```python
from build123d import *

# Parameters (mm, degrees)
SKETCH_2_R      = 1.25
EXTRUDE_1_DEPTH = 1.8


with BuildPart() as part:
    # Эскиз2 → Бобышка-Вытянуть1 (new body)
    with BuildSketch(Plane(origin=(0, 0, 0), x_dir=(1, 0, 0), z_dir=(0, 1, 0))):
        with Locations(Location((0, 0, 0), (0, 0, 270))):
            Circle(SKETCH_2_R)
    extrude(amount=-EXTRUDE_1_DEPTH)

    # Эскиз4 → Повернуть1 (revolve)
    with BuildSketch(Plane.XY, mode=Mode.PRIVATE) as revolve_1_sk:
        with BuildLine():
            Line((0, 0), (0, 1))
            Line((0, 1), (4, 1))
            ThreePointArc((4, 1), (3.323810781, 0.850092459), (2.774328891, 0.428460175))
            Line((2.774328891, 0.428460175), (2.654597544, 0.285769912))
            ThreePointArc((2.654597544, 0.285769912), (2.379856599, 0.07495377), (2.041761989, 0))
            Line((2.041761989, 0), (1.25, 0))
            Line((1.25, 0), (0, 0))
        make_face()
    revolve(revolve_1_sk.sketch.rotate(Axis((0, 0, 0), (0, 1, 0)), 90), axis=Axis((0, 0, 0), (0, 1, 0)))


solid = part.part
```
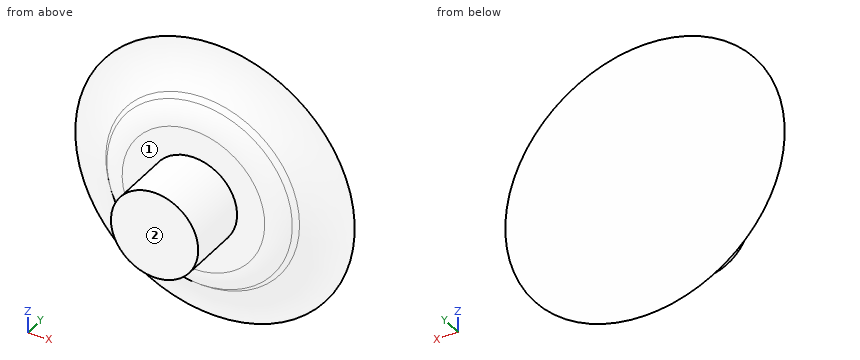
Work out the finished part from the listing and answer in its coordinate system (mm). Face numbers are marked on the shaded views. A direction names the side the tool comes from. Give positions to 0.01 mm unless a question says otherwise; leave off trailing zeros. Order: outer loops, then holes, each group sorted by start corner. A loop starts at its lowest first (then second) coordinate and runs counter-clockwise, first axis right, second up. Notation, with made-up numbers: (79, -27) -> (131, -27) arc R18 ccw to (131, 6) -> close; hole circle Ø2 at (-28.75, -16). An arc over 180 degrees is marked (long way). Answer as CSV lines item,"result". Start each with the question number.
(1) Section B-B, the plane z = 0 is taken. Write down the section's boundary in (x, y), plus the area to 3 significant figures.
(2) This flat-tipped pin is pushed along its axis until it touches: pin 1 Ø1.5 at (y, z) = (-1, -1.5) entering from -X. Where does it stop, or does it pass through?
(3) Which of the six approach directions +Z, -Z, +X, -X, +Y, -Y give full straight-line access (tool end or side, diameter ignored) to the marked faces 1 and 2?
(4) Section A-A, the plane x = 0 is taken. Write down the section's boundary in (y, z), plus the area to 3 significant figures.
(5) Section C-C, the plane y = 0.7 is taken. Write down the section's boundary in (x, z), plus the area to 3 significant figures.
(6) Section D-D, the plane y = -0.3 is taken. Write down the section's boundary in (x, z), plus the area to 3 significant figures.
(7) Consider line 1 along Z through (x, y) = (1.25, 0.6); line 2 along Y through (x, z) = (0.25, -3); line 3 along Z through (x, y) = (-1, 0.6). Determine where each line is inside the solid, lowest interval first.
Entries:
1,outline,"(-4, 1) arc R1.6 cw to (-2.77, 0.43) -> (-2.65, 0.29) arc R0.8 ccw to (-2.04, 0) -> (-1.25, 0) -> (-1.25, -1.8) -> (1.25, -1.8) -> (1.25, 0) -> (2.04, 0) arc R0.8 ccw to (2.65, 0.29) -> (2.77, 0.43) arc R1.6 cw to (4, 1) -> close"
1,area,"10.3 mm²"
2,pin 1,"x = -1"
3,face 1,"-Y"
3,face 2,"+Z, -Z, +X, -X, -Y"
4,outline,"(-1.8, -1.25) -> (0, -1.25) -> (0, -2.04) arc R0.8 ccw to (0.29, -2.65) -> (0.43, -2.77) arc R1.6 cw to (1, -4) -> (1, 4) arc R1.6 cw to (0.43, 2.77) -> (0.29, 2.65) arc R0.8 ccw to (0, 2.04) -> (0, 1.25) -> (-1.8, 1.25) -> close"
4,area,"10.3 mm²"
5,outline,"circle Ø6.13 at (0, 0)"
5,area,"29.6 mm²"
6,outline,"circle Ø2.5 at (0, 0)"
6,area,"4.91 mm²"
7,line 1,"-2.66 to 2.66"
7,line 2,"0.66 to 1"
7,line 3,"-2.77 to 2.77"
